Model file for the job. Use its own axes, mm. Face numbers are marked on the shaded views. A direction names the side the tool comes from. Coordinates: 2 decimals unless noted, no trailing zeros. Loops run counter-clockwise (first coordinate to the right, second up) from the corner with the lowest first, then second, coordinate; pieces in that order, holes last. Notation, with made-up numbers: (44, 67.5) -> (92, 67.5) arc R29 cw to (92, 104.5) -> close; hole circle Ø3 at (-19.5, 75). An arc over 180 degrees is marked (long way). Use one line per item in the form item = value.
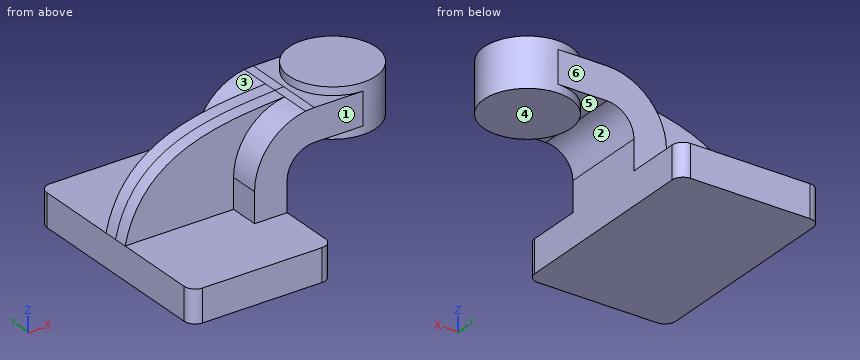
```python
from build123d import *

# Parameters (mm, degrees)
F1_DEPTH = 63.5
F2_DEPTH = 25.4
F3_DEPTH = 7.9375
F5_R     = 6.35


with BuildPart() as f1:
    # F0 (on Front) → F1 (new body, symmetric)
    with BuildSketch(Plane.XZ):
        Polygon((41.275, -9.525), (41.275, 9.525), (22.225, 9.525), (-41.275, 9.525), (-41.275, -9.525), align=None)
    extrude(amount=F1_DEPTH, both=True)

    # F0 (on Front) → F2 (join, symmetric)
    with BuildSketch(Plane.XZ):
        with BuildLine():
            Line((22.225, 9.525), (41.275, 9.525))
            Line((41.275, 9.525), (41.275, 27.0002))
            ThreePointArc((41.275, 27.0002), (45.92468, 38.22552), (57.15, 42.8752))
            Line((57.15, 42.8752), (60.325, 42.8752))
            Line((60.325, 42.8752), (60.325, 61.9252))
            Line((60.325, 61.9252), (57.15, 61.9252))
            add(Edge.make_bspline(
                [(52.001332, 61.543605), (53.732744, 61.669465), (55.450257, 61.795302), (57.15, 61.9252)],
                knots=[106.66287, 106.66287, 106.66287, 106.66287, 111.504536, 111.504536, 111.504536, 111.504536], degree=3))
            ThreePointArc((52.001332, 61.543605), (30.696523, 49.803033), (22.225, 27.0002))
            Line((22.225, 27.0002), (22.225, 9.525))
        make_face()
        Polygon((60.325, 61.9252), (60.325, 42.8752), (73.367334, 42.8752), (85.725, 42.8752), (85.725, 61.9252), (73.367334, 61.9252), align=None)
    extrude(amount=F2_DEPTH, both=True)

    # F0 (on Front) → F3 (join, symmetric)
    with BuildSketch(Plane.XZ):
        with BuildLine():
            Line((-41.275, 9.525), (22.225, 9.525))
            Line((22.225, 9.525), (22.225, 27.0002))
            ThreePointArc((22.225, 27.0002), (30.696523, 49.803033), (52.001332, 61.543605))
            add(Edge.make_bspline(
                [(-41.275, 9.525), (-31.030923, 55.987171), (13.857985, 58.770894), (52.001332, 61.543605)],
                knots=[0, 0, 0, 0, 106.66287, 106.66287, 106.66287, 106.66287], degree=3))
        make_face()
    extrude(amount=F3_DEPTH, both=True)

    # F0 (on Front) → F4 (revolve)
    with BuildSketch(Plane.XZ):
        Polygon((85.725, 42.8752), (85.725, 38.1), (111.125, 38.1), (111.125, 66.675), (85.725, 66.675), (85.725, 61.9252), align=None)
    revolve(axis=Axis((85.725, 0, 52.3875), (0, 0, 1)))

    # F5
    f5_edges = [f1.edges().sort_by_distance(p)[0] for p in [
        (41.275, -63.5, 0),
        (-41.275, -63.5, 0),
        (-41.275, 63.5, 0),
        (41.275, 63.5, 0),
    ]]
    fillet(f5_edges, radius=F5_R)


solid = f1.part
```
Q1. Pin check, flat tips, straight feed: pin 1 Ø10 at (x, z) = (50.5, 29.5) entering from -Y; pin 2 Ø19 at (y, z) = (-15, 21.5) entering from -X; pin 3 Ø15.5 at (x, z) = (17.5, 34) entering from -Y; pin 4 Ø15.5 at (x, z) = (66.5, 45) entering from +Y. Stop position of each tip, or through.
Result:
pin_1 = through
pin_2 = -39.81
pin_3 = -25.4
pin_4 = 25.4
Q2. Mould opens along X. For the marked faces 1, 2 and 3 say: released by +X, released by -X, zero draft, split by the parting line, or undercut.
Result:
face_1 = zero draft
face_2 = undercut
face_3 = released by -X
Q3. Which spindle directions (+Z, -Z, +X, -X, +Y, -Y) get a long thin tool onto all of the face, cutting with end or side? Do the marked faces 4, 5 and 6. Say none if no direction does.
Result:
face_4 = -Z, +X, +Y, -Y
face_5 = -Z
face_6 = +Z, +X, -X, +Y
Q4. Band-saw the part on A-A, the plane x = 65. Write the cut outline in (y, z) (1 decimal), and give its area (3 significant figures).
Result:
outline = (-25.4, 42.9) -> (-14.7, 42.9) -> (-14.7, 38.1) -> (14.7, 38.1) -> (14.7, 42.9) -> (25.4, 42.9) -> (25.4, 61.9) -> (14.7, 61.9) -> (14.7, 66.7) -> (-14.7, 66.7) -> (-14.7, 61.9) -> (-25.4, 61.9) -> close
area = 1,250 mm2
Q5. Wall check: line 1 along Z through (x, y) = (8, -15) (3 decimals); line 2 along Y through (x, z) = (38, 29.5); line 3 along Z through (x, y) = (73, 9) (3 decimals). Give the ranges that are in metal, low to high.
Result:
line_1 = -9.525 to 9.525
line_2 = -25.4 to 25.4
line_3 = 38.1 to 66.675
